Could you check a few things on this model? Use its own coordinates, in mm. A direction names the side the tool comes from. Coordinates: 2 decimals unless noted, no trailing zeros. Order: outer loops, then holes, each group sorted by start corner. A loop starts at its lowest first (then second) coordinate and runs counter-clockwise, first axis right, second up. Notation, with made-up numbers: (-17, 59) -> (20, 59) arc R21 ccw to (20, 69) -> close; hole circle Ø7 at (18, 36.5). An arc over 180 degrees is marked (long way). Use a Markdown table: item, result. Add a question column.
1) If we section it at B-B (x = 1): Write out the boundary of the cut face in (y, z) (3 decimals), plus the area to 3 significant figures.
2) If we section it at A-A (y = 7.25): Write out the boundary of the cut face in (x, z) (1 decimal), plus the area to 3 significant figures.
3) If we section it at C-C (x = 6.75): Write out the boundary of the cut face in (y, z) (1 decimal).
4) Will these pins go through, and if not, where does the flat tip stop? pin 1 Ø1.3 at (y, z) = (8, 4) entering from +X (3 decimals); pin 2 Ø5.5 at (y, z) = (7.5, -4) entering from +X; pin 3 Ø1.9 at (y, z) = (-1, 0) entering from -X.
5) Thinking about a two-plate mould opening in Z: for faces 5 (the flat face through (-3.175, -7.1, 4.4)), 6 (the cylindrical face through (-6, 5, 0)), 7 (the flat face through (-1.57, -7.06, -3.63)), which applies, +Z half, -Z half, draft (parallel to the pull), parting line (faces both ways), or undercut?
6) If I drill on L1, parallel to Z at x = -4.5, y = 0; L2, parallel to X at y = 7.75, z = -0.25; L3, parallel to Z at x = 12, y = -1.25, over which ranges is the centre line in solid material (lowest first)? Write a range as [from, to].
7) Which directions (+Z, -Z, +X, -X, +Y, -Y) give clear straight access to the entire face, cutting with the end or side of a thin tool? Please do faces 1 (the conical face through (13.3, 2.1, 1.6)), 2 (the flat face through (-1.57, -6.67, 4.3)), 3 (the flat face through (-4.762, -5, 5)), 4 (the cylindrical face through (3.414, -2.957, -0.931)).
```python
from build123d import *

# Parameters (mm, degrees)
CHAMFER1_SIZE    = 0.79375
CHAMFER1_SIZE_2  = 3.175
EXTRUSION1_DEPTH = 3.175
ESQUISSE3_R      = 9.165435523
EXTRUSION2_DEPTH = 1.5875
ESQUISSE4_R      = 6.5786
THREAD1_DEPTH    = 4.7625
CHAMFER2_SIZE    = 0.79375
CHAMFER4_SIZE    = 1


with BuildPart() as part:
    # Esquisse1 → Revolution1 (revolve)
    with BuildSketch(Plane.XY, mode=Mode.PRIVATE) as revolution1_sk:
        Polygon((0, 1.703), (16, 1.703), (16, 3.1), (14, 3.1), (14, 2.465), (11.46, 3.1), (11.46, 2.465), (8.92, 3.1), (8.92, 2.465), (6.38, 3.1), (6.38, 2.465), (3.84, 3.1), (3, 3.1), (3, 2.465), (0, 2.465), align=None)
    revolve(revolution1_sk.sketch.rotate(Axis((0, 0, 0), (1, 0, 0)), 180), axis=Axis((0, 0, 0), (1, 0, 0)))

    # Chamfer1
    # the kernel refuses this chamfer: 3.175, 0.79375 mm, written as the material it takes off along each edge
    with BuildSketch(Plane(origin=(16, 0, 0), x_dir=(0, -1, 0), z_dir=(0, 0, 1))) as chamfer1_piece_1:
        Polygon((3.1 - CHAMFER1_SIZE, 0), (3.1, -CHAMFER1_SIZE_2), (3.1, 0), align=None)
    revolve(axis=Axis((16, 0, 0), (1, 0, 0)), mode=Mode.SUBTRACT)

    # Esquisse2 → Extrusion1 (add)
    with BuildSketch(Plane.ZY):
        Polygon((0.375877143, -9.157724865), (-7.742883803, -4.904381587), (-8.118760946, 4.253343278), (-0.375877143, 9.157724865), (7.742883803, 4.904381587), (8.118760946, -4.253343278), align=None)
    extrude(amount=EXTRUSION1_DEPTH)

    # Esquisse3 → Extrusion2 (add)
    with BuildSketch(Plane.ZY.offset(3.175)):
        with Locations(Location((0, 0, 0), (0, 0, 152.350375514))):
            Circle(ESQUISSE3_R)
    extrude(amount=EXTRUSION2_DEPTH)

    # Esquisse4 → Thread1 (add)
    with BuildSketch(Plane.ZY.offset(4.7625)):
        with Locations(Location((0, 0, 0), (0, 0, 180))):
            Circle(ESQUISSE4_R)
    extrude(amount=THREAD1_DEPTH)

    # Chamfer2
    chamfer2_edges = [part.edges().sort_by_distance(p)[0] for p in [
        (-9.525, 0, 6.5786),
    ]]
    chamfer(chamfer2_edges, length=CHAMFER2_SIZE)

    # Sketch1 → Cut-Revolve1 (revolve, cut)
    with BuildSketch(Plane(origin=(0, 0, 0), x_dir=(1, 0, 0), z_dir=(0, 1, 0)), mode=Mode.PRIVATE) as cut_revolve1_sk:
        Polygon((0, -1.703), (-2, -1.703), (-2, -5), (-9.525, -5), (-9.525, 0), (0, 0), align=None)
    revolve(cut_revolve1_sk.sketch.rotate(Axis((-9.525, 0, 0), (1, 0, 0)), 90), axis=Axis((-9.525, 0, 0), (1, 0, 0)), mode=Mode.SUBTRACT)

    # Chamfer4
    chamfer4_edges = [part.edges().sort_by_distance(p)[0] for p in [
        (-2, 1.703, 0),
    ]]
    chamfer(chamfer4_edges, length=CHAMFER4_SIZE)


solid = part.part
```
Answer sheet:
| question | item | result |
|---|---|---|
| 1 | outline | circle Ø4.93 at (0, 0); hole circle Ø3.406 at (0, 0) |
| 1 | area | 9.98 mm2 |
| 2 | outline | (-4.8, -5.6) -> (-3.2, -5.6) -> (-3.2, -3.4) -> (0, -3.4) -> (0, 3.3) -> (-3.2, 3.3) -> (-3.2, 5.6) -> (-4.8, 5.6) -> close |
| 2 | area | 38.9 mm2 |
| 3 | outline | circle Ø6 at (0, 0); hole circle Ø3.4 at (0, 0) |
| 4 | pin 1 | x = -3.175 |
| 4 | pin 2 | x = 0 |
| 4 | pin 3 | x = -1.25 |
| 5 | face 5 | draft |
| 5 | face 6 | undercut |
| 5 | face 7 | -Z half |
| 6 | L1 | [-9.17, -5], [5, 9.17] |
| 6 | L2 | [-4.76, 0] |
| 6 | L3 | [-2.69, -1.16], [1.16, 2.69] |
| 7 | face 1 | none |
| 7 | face 2 | +Z, +X, -Y |
| 7 | face 3 | -X |
| 7 | face 4 | +X |
